from build123d import *

# Parameters (mm, degrees)
F0_W     = 57.15
F0_H     = 19.05
F1_DEPTH = 19.05
F3_DEPTH = 19.05
F4_W     = 38.1
F4_H     = 19.05
F5_DEPTH = 19.05
F6_W     = 19.05
F6_H     = 19.05
F7_DEPTH = 19.05


with BuildPart() as f1:
    # F0 (on Front) → F1 (new body)
    with BuildSketch(Plane.XZ):
        with Locations((-68.856497, 35.426075)):
            Rectangle(F0_W, F0_H)
    extrude(amount=F1_DEPTH)

    # F2 (on face) → F3 (join)
    with BuildSketch(Plane.XZ.offset(19.05)):
        Polygon((-59.331497, 44.951075), (-78.381497, 44.951075), (-78.381497, 25.901075), (-59.331497, 25.901075), (-59.331497, 35.426075), align=None)
    extrude(amount=F3_DEPTH)

    # F4 (on face) → F5 (join)
    with BuildSketch(Plane(origin=(0, 0, 25.901075), x_dir=(1, 0, 0), z_dir=(0, 0, -1))):
        with Locations((-78.381497, 9.525)):
            Rectangle(F4_W, F4_H)
    extrude(amount=F5_DEPTH)

    # F6 (on face) → F7 (join)
    with BuildSketch(Plane(origin=(0, 0, 25.901075), x_dir=(1, 0, 0), z_dir=(0, 0, -1))):
        with Locations((-68.856497, 28.575)):
            Rectangle(F6_W, F6_H)
    extrude(amount=F7_DEPTH)


solid = f1.part
Geometry check sheet. Reference: the model listing, model coordinates, mm. A direction names the side the tool comes from. Coordinates: 2 decimals unless noted, no trailing zeros. Order: outer loops, then holes, each group sorted by start corner. A loop starts at its lowest first (then second) coordinate and runs counter-clockwise, first axis right, second up. Notation, with made-up numbers: (-12, 66.5) -> (14, 66.5) arc R12 cw to (14, 77.5) -> close; hole circle Ø5 at (-9, 0). An arc over 180 degrees is marked (long way). Use a Markdown table: item, result. Add a question column.
1. Set-up check for faces 1 (the face through (-50, -9, 25.901)), 2 (the face through (-69, -15, 44.951)), 3 (the face through (-78.381, -28, 26)), 4 (the face through (-50, -19.05, 36)): record each of +Z, -Z, +X, -X, +Y, -Y from which the full face is reachable in a straight line by a thin tool's end or side.
2. Go/stop test with flat-tipped pins: pin 1 Ø3 at (y, z) = (-6, 13) entering from +X; pin 2 Ø21 at (y, z) = (-30, 19.5) entering from -X; pin 3 Ø10 at (x, z) = (-52, 19.5) entering from -Y; pin 4 Ø15 at (x, z) = (-86, 30.5) entering from -Y. Record where each tip stops, or that it passes through.
3. Cross-section at B-B (y = -15.5). Enter the section's corners in (x, z).
4. Material ranges on L1, parallel to X at y = -6.5, z = 19; L2, parallel to Z at x = -56.5, y = -11.5; L3, parallel to Y at x = -95, z = 37, recorded low to high.
5. Cross-section at D-D (z = 40). Enter the section's corners in (x, y), and give its area (3 significant figures).
6. Cross-section at C-C (x = -47). Enter the section's corners in (y, z), and give its area (3 significant figures).
7. Cross-section at A-A (z = 18.5). Enter the section's corners in (x, y).
Filled sheet:
| question | item | result |
|---|---|---|
| 1 | face 1 | -Z, +X, +Y, -Y |
| 1 | face 2 | +Z, +X, -X, +Y, -Y |
| 1 | face 3 | +Z, -Z, -X, -Y |
| 1 | face 4 | +Z, -Z, +X, -Y |
| 2 | pin 1 | x = -59.33 |
| 2 | pin 2 | x = -78.38 |
| 2 | pin 3 | through |
| 2 | pin 4 | y = -19.05 |
| 3 | outline | (-97.43, 6.85) -> (-59.33, 6.85) -> (-59.33, 25.9) -> (-40.28, 25.9) -> (-40.28, 44.95) -> (-97.43, 44.95) -> close |
| 4 | L1 | -97.43 to -59.33 |
| 4 | L2 | 25.9 to 44.95 |
| 4 | L3 | -19.05 to 0 |
| 5 | outline | (-97.43, -19.05) -> (-78.38, -19.05) -> (-78.38, -38.1) -> (-59.33, -38.1) -> (-59.33, -19.05) -> (-40.28, -19.05) -> (-40.28, 0) -> (-97.43, 0) -> close |
| 5 | area | 1,450 mm2 |
| 6 | outline | (-19.05, 25.9) -> (0, 25.9) -> (0, 44.95) -> (-19.05, 44.95) -> close |
| 6 | area | 363 mm2 |
| 7 | outline | (-97.43, -19.05) -> (-78.38, -19.05) -> (-78.38, -38.1) -> (-59.33, -38.1) -> (-59.33, 0) -> (-97.43, 0) -> close |
